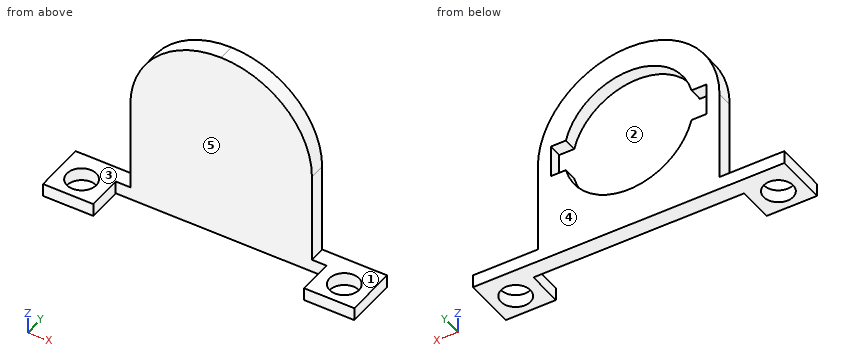
from build123d import *

# Parameters (mm, degrees)
SKETCH_1_W          = 96
SKETCH_1_H          = 16
EXTRUDE_1_DEPTH     = 4
SKETCH_2_W          = 56
SKETCH_2_H          = 5
EXTRUDE_2_DEPTH     = 56
SKETCH_3_W          = 65
SKETCH_3_H          = 11
CUT_EXTRUDE_1_DEPTH = 50
SKETCH_4_R          = 4.55
CUT_EXTRUDE_2_DEPTH = 75.188947964
FILLET_1_R          = 28
CUT_EXTRUDE_3_DEPTH = 4.1


with BuildPart() as part:
    # 스케치1 → 보스-돌출1 (new body)
    with BuildSketch(Plane.XY):
        Rectangle(SKETCH_1_W, SKETCH_1_H)
    extrude(amount=EXTRUDE_1_DEPTH)

    # 스케치2 → 보스-돌출2 (add)
    with BuildSketch(Plane.XY.offset(4)):
        with Locations((0, 5.5)):
            Rectangle(SKETCH_2_W, SKETCH_2_H)
    extrude(amount=EXTRUDE_2_DEPTH)

    # 스케치3 → 컷-돌출1 (cut)
    with BuildSketch(Plane.XY.offset(4)):
        with Locations((0, -2.5)):
            Rectangle(SKETCH_3_W, SKETCH_3_H)
    extrude(amount=-CUT_EXTRUDE_1_DEPTH, mode=Mode.SUBTRACT)

    # 스케치4 → 컷-돌출2 (cut, through all)
    with BuildSketch(Plane.XY.offset(4)):
        with Locations((40.5, -1)):
            Circle(SKETCH_4_R)
        with Locations((-40.5, -1)):
            Circle(SKETCH_4_R)
    extrude(amount=-CUT_EXTRUDE_2_DEPTH, mode=Mode.SUBTRACT)

    # 필렛1
    fillet_1_edges = [part.edges().sort_by_distance(p)[0] for p in [
        (-28, 5.5, 60),
        (28, 5.5, 60),
    ]]
    fillet(fillet_1_edges, radius=FILLET_1_R - 0.0001)  # a hair under: the kernel refuses the full size

    # 스케치5 → 컷-돌출3 (cut)
    with BuildSketch(Plane(origin=(0, 8, 0), x_dir=(1, 0, 0), z_dir=(0, 1, 0))):
        with BuildLine():
            Line((-19.364916731, -27), (-16, -27))
            Line((-16, -27), (-16, -37))
            Line((-16, -37), (-19.364916731, -37))
            ThreePointArc((-19.364916731, -37), (0, -52), (19.364916731, -37))
            Line((19.364916731, -37), (16, -37))
            Line((16, -37), (16, -27))
            Line((16, -27), (19.364916731, -27))
            ThreePointArc((19.364916731, -27), (0, -12), (-19.364916731, -27))
        make_face()
        with BuildLine():
            ThreePointArc((20, -32), (19.840593925, -29.47991415), (19.364916731, -27))
            Line((19.364916731, -27), (16, -27))
            Line((16, -27), (16, -37))
            Line((16, -37), (19.364916731, -37))
            ThreePointArc((19.364916731, -37), (19.840593925, -34.52008585), (20, -32))
        make_face()
        with BuildLine():
            Line((24, -27), (19.364916731, -27))
            ThreePointArc((19.364916731, -27), (19.840593925, -29.47991415), (20, -32))
            ThreePointArc((20, -32), (19.840593925, -34.52008585), (19.364916731, -37))
            Line((19.364916731, -37), (24, -37))
            Line((24, -37), (24, -27))
        make_face()
        with BuildLine():
            Line((-16, -37), (-16, -27))
            Line((-16, -27), (-19.364916731, -27))
            ThreePointArc((-19.364916731, -27), (-20, -32), (-19.364916731, -37))
            Line((-19.364916731, -37), (-16, -37))
        make_face()
        with BuildLine():
            ThreePointArc((-19.364916731, -37), (-20, -32), (-19.364916731, -27))
            Line((-19.364916731, -27), (-24, -27))
            Line((-24, -27), (-24, -37))
            Line((-24, -37), (-19.364916731, -37))
        make_face()
    extrude(amount=-CUT_EXTRUDE_3_DEPTH, mode=Mode.SUBTRACT)


solid = part.part
Read the model definition and answer for the solid it produces. Units are mm, in the model's axes. Face numbers are marked on the shaded views. A direction names the side the tool comes from. Coordinates: 2 decimals unless noted, no trailing zeros. Order: outer loops, then holes, each group sorted by start corner. A loop starts at its lowest first (then second) coordinate and runs counter-clockwise, first axis right, second up. Notation, with made-up numbers: (33.25, 3) -> (74.25, 3) arc R26 cw to (74.25, 36) -> close; hole circle Ø4 at (-32, 29.25). An arc over 180 degrees is marked (long way). Answer as a JSON object with one key per item and string values.
1) A cutting plane is placed at C-C, the plane z = 41.5. Determine the outline of the cut face in (x, y), plus the area to 3 significant figures.
Model answer:
{"outline": "(-26.34, 3) -> (26.34, 3) -> (26.34, 8) -> (17.6, 8) -> (17.6, 3.9) -> (-17.6, 3.9) -> (-17.6, 8) -> (-26.34, 8) -> close", "area": "119 mm²"}
2) A tool of negligible diameter and unlimited length cuts with its end or side. For the marked faces 3, 4 and 5, from which of +Z, -Z, +X, -X, +Y, -Y can it reach the whole face along a straight path? Write none if from no direction.
Model answer:
{"face 3": "+Z, -X, +Y, -Y", "face 4": "+Z, -Z, +X, -X, +Y", "face 5": "+Z, -Z, -Y"}
3) Consider line 1 along X through (y, z) = (4.5, 32); line 2 along X through (y, z) = (6.5, 46.5); line 3 along Y through (x, z) = (-40, 2). Determine where each line is inside the solid, lowest interval first. Write a range as from..to.
Model answer:
{"line 1": "x = -28..-24, 24..28", "line 2": "x = -23.95..-13.77, 13.77..23.95", "line 3": "y = -8..-5.52, 3.52..8"}
4) A cutting plane is placed at A-A, the plane y = -1. Determine the outline of the cut face in (x, z).
Model answer:
{"outline": "(-48, 0) -> (-45.05, 0) -> (-45.05, 4) -> (-48, 4) -> close; (-35.95, 0) -> (-32.5, 0) -> (-32.5, 4) -> (-35.95, 4) -> close; (32.5, 0) -> (35.95, 0) -> (35.95, 4) -> (32.5, 4) -> close; (45.05, 0) -> (48, 0) -> (48, 4) -> (45.05, 4) -> close"}
5) The mould has two halves that part along X. Classify the marked faces 1 and 2: released by +X, released by -X, zero draft, split by the parting line, or undercut.
Model answer:
{"face 1": "zero draft", "face 2": "undercut"}
6) Each of these flat-tipped pins is pushed along its axis until it touches: pin 1 (1.2 mm diameter, centred on x = 22.5, y = 5.5, fed in from +Z); pin 2 (1.5 mm diameter, centred on x = 25, y = 2.5, fed in from +Z); pin 3 (12 mm diameter, centred on x = -26.5, z = 38.5, fed in from -Y); pin 4 (1.2 mm diameter, centred on x = 22.5, y = 5.5, fed in from -Z). Where does it stop, or does it pass through?
Model answer:
{"pin 1": "stops at z = 49.45", "pin 2": "stops at z = 45.66", "pin 3": "stops at y = 3", "pin 4": "stops at z = 0"}
7) A cutting plane is placed at D-D, the plane x = 34. Determine the outline of the cut face in (y, z), plus the area to 3 significant figures.
Model answer:
{"outline": "(-8, 0) -> (8, 0) -> (8, 4) -> (-8, 4) -> close", "area": "64.0 mm²"}
8) A cutting plane is placed at B-B, the plane x = -40.5. Determine the outline of the cut face in (y, z), plus the area to 3 significant figures.
Model answer:
{"outline": "(-8, 0) -> (-5.55, 0) -> (-5.55, 4) -> (-8, 4) -> close; (3.55, 0) -> (8, 0) -> (8, 4) -> (3.55, 4) -> close", "area": "27.6 mm²"}
